The listing builds one solid part. Answer for the finished solid, in the listing's coordinates (mm). A direction names the side the tool comes from. Round coordinates to 2 decimals unless told otherwise and drop trailing zeros. Write each loop counter-clockwise with the first axis right and the second up, starting at its lowest first coordinate (ties: lowest second). Pieces come first, ordered by that corner, then holes. Notation, with made-up numbers: (43, 53.25) - (101, 53.25) arc R18 cw to (101, 77.25) - close; hole circle Ø10 at (33, 56). An arc over 180 degrees is marked (long way). Return JSON: item names as keys, results as strings. Group by question number.
from build123d import *

# Parameters (mm, degrees)
SKETCH1_W           = 152.4
SKETCH1_H           = 57.15
BOSS_EXTRUDE1_DEPTH = 6.35
CUT_EXTRUDE1_DEPTH  = 7.35
CUT_EXTRUDE2_DEPTH  = 58.15
SKETCH4_W           = 3.175
SKETCH4_H           = 4.7625
CUT_EXTRUDE3_DEPTH  = 153.4
SKETCH5_W           = 3.175
SKETCH5_H           = 3.2512
CUT_EXTRUDE4_DEPTH  = 153.4
SKETCH6_R           = 2.3876
CUT_EXTRUDE5_DEPTH  = 5.08


with BuildPart() as part:
    # Sketch1 → Boss-Extrude1 (new body)
    with BuildSketch(Plane.XY):
        with Locations((76.2, 28.575)):
            Rectangle(SKETCH1_W, SKETCH1_H)
    extrude(amount=-BOSS_EXTRUDE1_DEPTH)

    # Sketch2 → Cut-Extrude1 (cut, through all)
    with BuildSketch(Plane.XY):
        with BuildLine():
            Line((32.5501, 30.1625), (119.8626, 30.1625))
            ThreePointArc((119.8626, 30.1625), (121.4501, 28.575), (119.8626, 26.9875))
            Line((119.8626, 26.9875), (32.5501, 26.9875))
            ThreePointArc((32.5501, 26.9875), (30.9626, 28.575), (32.5501, 30.1625))
        make_face()
    extrude(amount=-CUT_EXTRUDE1_DEPTH, mode=Mode.SUBTRACT)

    # Sketch3 → Cut-Extrude2 (cut, through all)
    with BuildSketch(Plane(origin=(0, 57.15, 0), x_dir=(1, 0, 0), z_dir=(0, 1, 0))):
        Polygon((152.4, 0), (146.05, 6.35), (152.4, 6.35), align=None)
        Polygon((0, 0), (6.35, 6.35), (0, 6.35), align=None)
    extrude(amount=-CUT_EXTRUDE2_DEPTH, mode=Mode.SUBTRACT)

    # Sketch4 → Cut-Extrude3 (cut, through all)
    with BuildSketch(Plane(origin=(0, 0, 0), x_dir=(0, 0, -1), z_dir=(1, 0, 0))):
        with Locations((4.7625, 43.97375)):
            Rectangle(SKETCH4_W, SKETCH4_H)
    extrude(amount=CUT_EXTRUDE3_DEPTH, mode=Mode.SUBTRACT)

    # Sketch5 → Cut-Extrude4 (cut, through all)
    with BuildSketch(Plane(origin=(0, 0, 0), x_dir=(0, 0, -1), z_dir=(1, 0, 0))):
        with Locations((4.7625, 6.3881)):
            Rectangle(SKETCH5_W, SKETCH5_H)
    extrude(amount=CUT_EXTRUDE4_DEPTH, mode=Mode.SUBTRACT)

    # Sketch6 → Cut-Extrude5 (cut)
    with BuildSketch(Plane(origin=(0, 0, -6.35), x_dir=(-1, 0, 0), z_dir=(0, 0, -1))):
        with Locations((-9.652, 49.911)):
            Circle(SKETCH6_R)
    extrude(amount=-CUT_EXTRUDE5_DEPTH, mode=Mode.SUBTRACT)


solid = part.part
(1) Find section B-B (z = -4.5). State how many separate pieces and enclosed holes the cut face has, plus the area to 3 significant figures.
(2) Determine the mould class of faces 6 (the flat face through (3, 29, -3)), 7 (the flat face through (10, 50, -1.27)), 8 (the flat face through (75, 57.15, -3)), 9 (the flat face through (75, 0, -3)) for opening direction Y: +Y half, -Y half, draft (parallel to the pull), parting line (faces both ways), or undercut.
(3) Flat-ended cylindrical pins translate along their axes: pin 1 (1 mm diameter, centred on y = 48, z = -1, fed in from +X); pin 2 (3 mm diameter, centred on y = 9.5, z = -5.5, fed in from +X); pin 3 (2 mm diameter, centred on y = 23.5, z = -2.5, fed in from -X). Find the tip coordinate at first contact, or state that the pin passes through.
(4) For faces 1 (the flat face through (75, 46.355, -5)), 2 (the cylindrical face through (11.412, 51.525, -3.846)), 3 (the cylindrical face through (30.963, 28.54, -3.131)), 4 (the flat face through (75, 35, 0)), 5 (the flat face through (75, 52, -6.35)), determine the directions among +Z, -Z, +X, -X, +Y, -Y from which every point of the face is accessible in a straight line to the end or side of a thin tool.
(5) Find section D-D (y = 45). Write down the section's boundary in (x, z) (3 decimals), plus the area to 3 significant figures.
(6) Consider line 1 (Y direction, x = 103, z = -0.5); line 2 (X direction, y = 28, z = -6); line 3 (X direction, y = 51, z = -4.25). Determine where each line is inside the solid, lowest interval first.
Check sheet entries:
{
 "1": {"separate pieces": "3", "enclosed holes": "2", "area": "6,740 mm^2"},
 "2": {"face 6": "draft", "face 7": "undercut", "face 8": "+Y half", "face 9": "-Y half"},
 "3": {"pin 1": "stops at x = 151.9", "pin 2": "stops at x = 148.4", "pin 3": "stops at x = 1.5"},
 "4": {"face 1": "-Z, +X, -X", "face 2": "-Z", "face 3": "+Z, -Z", "face 4": "+Z, +X, -X, +Y, -Y", "face 5": "-Z, +X, -X, +Y, -Y"},
 "5": {"outline": "(0, 0) - (3.175, -3.175) - (149.225, -3.175) - (152.4, 0) - close", "area": "474 mm^2"},
 "6": {"line 1": "y = 0 to 26.99, 30.16 to 57.15", "line 2": "x = 6 to 31.07, 121.34 to 146.4", "line 3": "x = 4.25 to 7.53, 11.78 to 148.15"}
}
